Autodesk Inventor part; units mm, degrees
ref_plane "YZ Plane" through (0, 0, 0) normal (1, 0, 0) x (0, 1, 0)
ref_plane "XZ Plane" through (0, 0, 0) normal (0, 1, 0) x (-1, 0, 0)
ref_plane "XY Plane" through (0, 0, 0) normal (0, 0, 1) x (1, 0, 0)
sketch "Sketch1" plane through (0, 0, 0) normal (0, 0, 1) x (1, 0, 0)
  line L0 (-28, 25) -> (28, 25)
  line L1 (28, 25) -> (28, 15)
  line L2 (28, 15) -> (14, 15)
  line L3 (14, 15) -> (14, -15)
  line L4 (14, -15) -> (10, -15)
  line L5 (10, -15) -> (10, 15)
  line L6 (10, 15) -> (-10, 15)
  line L7 (-10, 15) -> (-10, -15)
  line L8 (-10, -15) -> (-14, -15)
  line L9 (-14, -15) -> (-14, 15)
  line L10 (-14, 15) -> (-28, 15)
  line L11 (-28, 15) -> (-28, 25)
  point P0 (0, 0)
  point P1 (0, 25)
  point P2 (0, 15)
  point P3 (10, 0)
  dimension "d0" = 20
  dimension "d1" = 30
  dimension "d2" = 4
  dimension "d3" = 4
  dimension "d4" = 14
  dimension "d5" = 10
extrude "Extrusion1" add sketch "Sketch1" along normal mid plane 15
sketch "Sketch2" plane through (-28, 25, 7.5) normal (0, 1, 0) x (1, 0, 0)
  circle A0 centre (6, 7.5) radius 2.6
  circle A1 centre (50, 7.5) radius 2.6
  line L0 (0, 15) -> (0, 0)
  line L1 (56, 0) -> (56, 15)
  point P0 (28, 7.5)
  dimension "d8" = 5.2
  dimension "d9" = 6
  dimension "d10" = 6
extrude "Extrusion2" cut sketch "Sketch2" against normal up to next
sketch "Sketch3" plane through (-28, 15, 7.5) normal (0, -1, 0) x (1, 0, 0)
  circle A0 centre (6, -7.5) radius 2.6
  circle A1 centre (50, -7.5) radius 2.6
  line L0 (1.9, -10.2201) -> (1.9, -4.7799)
  line L1 (1.9, -4.7799) -> (6, -3.05)
  line L2 (6, -3.05) -> (10.1, -4.7799)
  line L3 (10.1, -4.7799) -> (10.1, -10.2201)
  line L4 (14, 0) -> (14, -15)
  line L5 (10.1, -10.2201) -> (6, -11.95)
  line L6 (6, -11.95) -> (1.9, -10.2201)
  point P0 (28, -7.5)
  point P1 (1.9, -7.5)
  dimension "d13" = 8.2
  dimension "d22" = 8.9
  dimension "d23" = 8.2
extrude "Extrusion3" cut sketch "Sketch3" against normal blind 5 contours L0 L1 L2 L3 L5 L6
mirror "Mirror1" about plane through (0, 0, 0) normal (1, 0, 0) of "Extrusion3"
sketch "Sketch4" plane through (14, -15, 7.5) normal (1, 0, 0) x (0, 0, -1)
  circle A0 centre (10, 10) radius 2.1
  line L0 (0, 0) -> (15, 0)
  point P0 (7.5, 15)
  point P1 (7.5, 0)
  point P2 (7.5, 0)
  dimension "d24" = 4.2
  dimension "d25" = 10
extrude "Extrusion4" cut sketch "Sketch4" against normal up to surface (28 mm away)
fillet "Fillet1" radius 5 4 edges at (-28, 20, 7.5) (-28, 20, -7.5) (28, 20, 7.5) (28, 20, -7.5)
chamfer "Chamfer1" distance 3 angle 45 2 edges at (-14, 15, 0) (14, 15, 0)
sketch "Sketch8" plane through (0, 0, 7.5) normal (0, 0, 1) x (1, 0, 0)
  line L0 (-10, 15) -> (10, 15)
  line L1 (10, 15) -> (10, -15)
  line L2 (10, -15) -> (-10, -15)
  line L3 (-10, -15) -> (-10, 15)
  point P0 (0, 0)
extrude "Extrusion7" add sketch "Sketch8" against normal blind 3
sketch "Sketch9" plane through (0, 0, -7.5) normal (0, 0, -1) x (-1, 0, 0)
  line L0 (-10, 5) -> (10, 5)
  line L1 (10, -15) -> (14, -15)
  line L2 (-10, 5) -> (-10, 15)
  line L3 (-10, 15) -> (10, 15)
  line L4 (10, 15) -> (10, 5)
  point P0 (0, 0)
  dimension "d44" = 20
extrude "Extrusion8" add sketch "Sketch9" against normal up to surface (12 mm away)
sketch "Sketch6" plane through (0, 0, 7.5) normal (0, 0, 1) x (1, 0, 0)
  line L0 (-3.25, 16) -> (3.25, 16)
  line L1 (3.25, 16) -> (10, 25)
  line L2 (28, 25) -> (-28, 25)
  line L3 (-3.25, 16) -> (-10, 25)
  line L4 (-10, 25) -> (10, 25)
  line L5 (-14, -15) -> (-10, -15)
  line L6 (-10, 5) -> (10, 5)
  line L7 (-3.25, 16) -> (-3.25, 9)
  line L8 (-3.25, 9) -> (3.25, 9)
  line L9 (3.25, 9) -> (3.25, 16)
  point P0 (0, 0)
  point P1 (0, 16)
  point P2 (0, 25)
  point P3 (-10, 15)
  point P4 (0, 25)
  point P5 (0, 25)
  dimension "d29" = 6.5
  dimension "d30" = 20
  dimension "d47" = 9
  dimension "d48" = 4
extrude "Extrusion5" cut sketch "Sketch6" against normal up to surface (15 mm away)
sketch "Sketch11" plane through (-3.25, 9, 7.5) normal (0, 1, 0) x (1, 0, 0)
  line L0 (13.25, 7.9) -> (13.25, 12.1)
  line L1 (17.25, 12.1) -> (17.25, 7.9)
  circle A0 centre (3.25, 10) radius 2.1
  point P0 (3.25, 7.5)
  point P1 (17.25, 10)
  dimension "d49" = 4.2
extrude "Extrusion9" cut sketch "Sketch11" against normal up to next
equation "\"d3\" = d2"
properties part number "holder-GT2-x-carriage-left"
CAD build for the part. Positions are in the model's coordinates, mm. A direction names the side the tool comes from. Give positions to 0.01 mm unless a question says otherwise; leave off trailing zeros. Loops run counter-clockwise (first coordinate to the right, second up) from the corner with the lowest first, then second, coordinate; pieces in that order, holes last. Notation, with made-up numbers: (8, -24) -> (14, -24) arc R22 cw to (14, 15) -> close; hole circle Ø3 at (-36, 81.25). An arc over 180 degrees is marked (long way). Use a Markdown table: item, result.
1. Slice it at B-B (y = 22). List the corners of the cut face in (x, z), plus the area to 3 significant figures.
Check result:
| item | result |
|---|---|
| outline | (-28, -2.5) arc R5 ccw to (-23, -7.5) -> (-7.75, -7.5) -> (-7.75, 7.5) -> (-23, 7.5) arc R5 ccw to (-28, 2.5) -> close; (7.75, -7.5) -> (23, -7.5) arc R5 ccw to (28, -2.5) -> (28, 2.5) arc R5 ccw to (23, 7.5) -> (7.75, 7.5) -> close; hole circle Ø5.2 at (-22, 0); hole circle Ø5.2 at (22, 0) |
| area | 544 mm^2 |
2. Which spindle directions (+Z, -Z, +X, -X, +Y, -Y) get a long thin tool onto all of the face, cutting with end or side? Do faces 4 (the flat face through (-10, -5, 0)), 5 (the flat face through (-26.1, 17, 0)), 6 (the flat face through (25, 15, -3.4)). Say none if no direction does.
Check result:
| item | result |
|---|---|
| face 4 | -Z, -Y |
| face 5 | -Y |
| face 6 | +Z, -Z, +X, -Y |
3. Mould opens along X. For faces 1 (the flat face through (-6.58, 20.44, 0.11)), 2 (the cylindrical face through (-11.97, -7.05, -2.04)), 3 (the flat face through (14, -1, 0)) say: pulls with the +X half, pulls with the -X half, needs draft (parallel to the pull), parting line crosses it, or undercut.
Check result:
| item | result |
|---|---|
| face 1 | undercut |
| face 2 | needs draft |
| face 3 | pulls with the +X half |
4. Slice it at A-A (x = 0). List the corners of the cut face in (y, z), plus the area to 3 significant figures.
Check result:
| item | result |
|---|---|
| outline | (-15, 4.5) -> (5, 4.5) -> (5, -0.4) -> (9, -0.4) -> (9, 7.5) -> (-15, 7.5) -> close; (5, -7.5) -> (9, -7.5) -> (9, -4.6) -> (5, -4.6) -> close |
| area | 103 mm^2 |
5. Slice it at D-D (y = 13). List the corners of the cut face in (x, z), plus the area to 4 significant figures.
Check result:
| item | result |
|---|---|
| outline | (-15, -7.5) -> (-3.25, -7.5) -> (-3.25, 7.5) -> (-15, 7.5) -> close; (3.25, -7.5) -> (15, -7.5) -> (15, 7.5) -> (3.25, 7.5) -> close |
| area | 352.5 mm^2 |
6. Flat gauge pins, fed straight in: pin 1 (3 mm diameter, centred on x = 4.5, z = 2, fed in from +Y); pin 2 (5.5 mm diameter, centred on x = 22, z = -1.5, fed in from -Y); pin 3 (5 mm diameter, centred on y = -5, z = -2.5, fed in from -X). Where does each tip first touch, or does it go through?
Check result:
| item | result |
|---|---|
| pin 1 | stops at y = 19.67 |
| pin 2 | stops at y = 15 |
| pin 3 | stops at x = -14 |
7. Wall check: L1, parallel to X at y = 16, z = 1.75; L2, parallel to X at y = 2, z = -5.25; L3, parallel to X at y = 11.5, z = -6.5. Give the ranges that are in metal, low to high. Write a range as [from, to].
Check result:
| item | result |
|---|---|
| L1 | x = [-28, -26.1], [-17.9, -3.25], [3.25, 17.9], [26.1, 28] |
| L2 | x = [-14, -10], [10, 14] |
| L3 | x = [-14, -3.25], [3.25, 14] |
8. Slice it at C-C (y = -5). List the corners of the cut face in (x, z), plus the area to 3 significant figures.
Check result:
| item | result |
|---|---|
| outline | (-14, -7.5) -> (-10, -7.5) -> (-10, -4.6) -> (-14, -4.6) -> close; (-14, -0.4) -> (-10, -0.4) -> (-10, 4.5) -> (10, 4.5) -> (10, -0.4) -> (14, -0.4) -> (14, 7.5) -> (-14, 7.5) -> close; (10, -7.5) -> (14, -7.5) -> (14, -4.6) -> (10, -4.6) -> close |
| area | 146 mm^2 |
